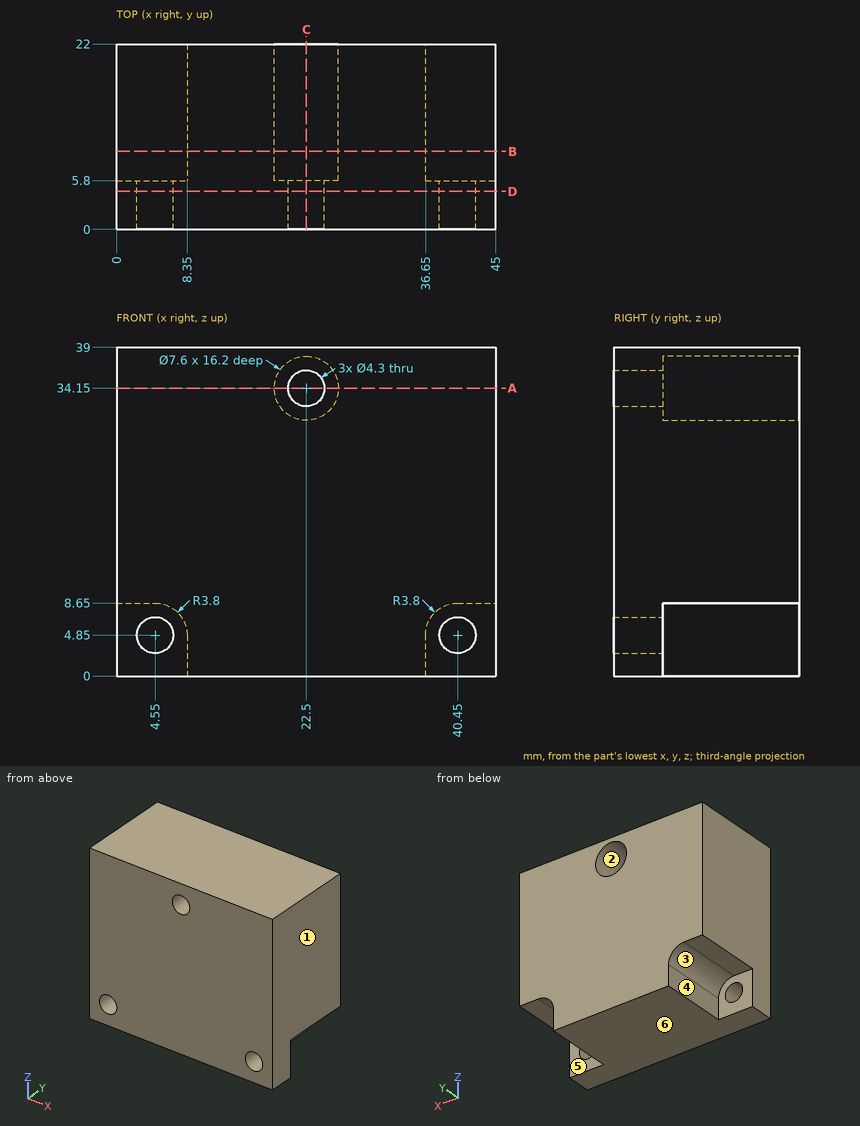
Verification items for this drawing (mm, ordinates from the low corner). A direction names the side the tool comes from. Coordinates: 2 decimals unless noted, no trailing zeros. Order: outer loops, then holes, each group sorted by start corner. A loop starts at its lowest first (then second) coordinate and runs counter-clockwise, first axis right, second up. Notation, with made-up numbers: M 27.25,-37 L 55.25,-37 A9 ccw 55.25,-26 Z; hole C 21.5,6.5 d4. An arc over 180 degrees is marked long. Use CSV: the item, a comma, the result in double quotes.
Item 1: Thickness scan on line 1 along X through (y, z) = (2.9, 4.85); line 2 along X through (y, z) = (17.75, 34.15); line 3 along Z through (x, y) = (22.5, 3.3). Record the ranges inside material, lowest first.
Returned:
line 1,"x = 0 to 2.4, 6.7 to 38.3, 42.6 to 45"
line 2,"x = 0 to 18.7, 26.3 to 45"
line 3,"z = 0 to 32, 36.3 to 39"
Item 2: Cross-section at D-D on y = 4.5. Record the cut outline in (x, z).
Returned:
outline,"M 0,0 L 45,0 L 45,39 L 0,39 Z; hole C 4.55,4.85 d4.3; hole C 22.5,34.15 d4.3; hole C 40.45,4.85 d4.3"
Item 3: Cross-section at B-B on y = 9.25. Record the cut outline in (x, z), then the cut area to 3 significant figures.
Returned:
outline,"M 0,8.65 L 4.55,8.65 A3.8 cw 8.35,4.85 L 8.35,0 L 36.65,0 L 36.65,4.85 A3.8 cw 40.45,8.65 L 45,8.65 L 45,39 L 0,39 Z; hole C 22.5,34.15 d7.6"
area,"1,570 mm2"
Item 4: Gauge pin test, flat ends, axial feed: pin 1 Ø3.5 at (x, z) = (4.55, 4.85) entering from -Y; pin 2 Ø2.5 at (x, z) = (3.5, 4) entering from +Y; pin 3 Ø10 at (x, z) = (22.5, 34.15) entering from -Y; pin 4 Ø5.5 at (y, z) = (10.5, 2.5) entering from -X. Record the tip position at first contact, or that the pin passes through.
Returned:
pin 1,"passes through"
pin 2,"stops at y = 5.8"
pin 3,"stops at y = 0"
pin 4,"stops at x = 8.33"
Item 5: Cross-section at C-C on x = 22.5. Record the cut outline in (y, z).
Returned:
outline,"M 0,0 L 22,0 L 22,30.35 L 5.8,30.35 L 5.8,32 L 0,32 Z; M 0,36.3 L 5.8,36.3 L 5.8,37.95 L 22,37.95 L 22,39 L 0,39 Z"
Item 6: Cross-section at A-A on z = 34.15. Record the cut outline in (x, y), then the cut area to 3 significant figures.
Returned:
outline,"M 0,0 L 20.35,0 L 20.35,5.8 L 18.7,5.8 L 18.7,22 L 0,22 Z; M 24.65,0 L 45,0 L 45,22 L 26.3,22 L 26.3,5.8 L 24.65,5.8 Z"
area,"842 mm2"
Item 7: Mould release check, pull along Z, two halves, no side actions. Record for the marked faces 1, 2 and 3: pulls with the +Z half, pulls with the -Z half, needs draft (parallel to the pull), parting line crosses it, or undercut.
Returned:
face 1,"needs draft"
face 2,"undercut"
face 3,"pulls with the -Z half"
Item 8: Tool access check on the marked faces 4, 5 and 6. Record the directions out of +Z, -Z, +X, -X, +Y, -Y that give a thin tool (end or side, any length) a straight path to the whole face; none if there is none.
Returned:
face 4,"-Z, -X, +Y"
face 5,"-Z, +X, +Y"
face 6,"-Z, +X, -X, +Y, -Y"
